from build123d import *

# Parameters (mm, degrees)
SZKIC2_W                    = 77
SZKIC2_H                    = 50
DODANIE_WYCI_GNI_CIE2_DEPTH = 4
SZKIC4_W                    = 50
SZKIC4_H                    = 46
WYTNIJ_WYCI_GNI_CIE1_DEPTH  = 4
SZKIC5_W                    = 77
SZKIC5_H                    = 4
DODANIE_WYCI_GNI_CIE3_DEPTH = 26
WYTNIJ_WYCI_GNI_CIE2_REACH  = 70.251
SZKIC6_R                    = 2
ZAOKR_GLENIE1_R             = 3
DODANIE_WYCI_GNI_CIE4_DEPTH = 4
DODANIE_WYCI_GNI_CIE5_DEPTH = 4
WYTNIJ_WYCI_GNI_CIE5_REACH  = 56.838
SZKIC9_R                    = 2


with BuildPart() as part:
    # Szkic2 → Dodanie-wyciągnięcie2 (new body)
    with BuildSketch(Plane(origin=(0, 0, 0), x_dir=(1, 0, 0), z_dir=(0, 1, 0))):
        Rectangle(SZKIC2_W, SZKIC2_H)
    extrude(amount=DODANIE_WYCI_GNI_CIE2_DEPTH)

    # Szkic4 → Wytnij-wyciągnięcie1 (cut)
    with BuildSketch(Plane.XZ):
        with Locations((0, -2)):
            Rectangle(SZKIC4_W, SZKIC4_H)
    extrude(amount=-WYTNIJ_WYCI_GNI_CIE1_DEPTH, mode=Mode.SUBTRACT)

    # Szkic5 → Dodanie-wyciągnięcie3 (add)
    with BuildSketch(Plane.XZ):
        with Locations((0, 23)):
            Rectangle(SZKIC5_W, SZKIC5_H)
    extrude(amount=DODANIE_WYCI_GNI_CIE3_DEPTH)

    # Szkic6 → Wytnij-wyciągnięcie2 (cut, up to next)
    with BuildSketch(Plane.XY.offset(25), mode=Mode.PRIVATE) as wytnij_wyci_gni_cie2_sk1:
        with Locations((26.5, -11)):
            Circle(SZKIC6_R)
    wytnij_wyci_gni_cie2_tool1 = extrude(wytnij_wyci_gni_cie2_sk1.sketch, amount=-WYTNIJ_WYCI_GNI_CIE2_REACH, mode=Mode.PRIVATE) & part.part
    # Szkic6 → Wytnij-wyciągnięcie2 (cut, up to next)
    with BuildSketch(Plane.XY.offset(25), mode=Mode.PRIVATE) as wytnij_wyci_gni_cie2_sk2:
        with Locations((-26.5, -11)):
            Circle(SZKIC6_R)
    wytnij_wyci_gni_cie2_tool2 = extrude(wytnij_wyci_gni_cie2_sk2.sketch, amount=-WYTNIJ_WYCI_GNI_CIE2_REACH, mode=Mode.PRIVATE) & part.part
    add(wytnij_wyci_gni_cie2_tool1.solids().sort_by_distance((26.5, -11, 25))[0], mode=Mode.SUBTRACT)
    add(wytnij_wyci_gni_cie2_tool2.solids().sort_by_distance((-26.5, -11, 25))[0], mode=Mode.SUBTRACT)

    # Zaokrąglenie1
    zaokr_glenie1_edges = [part.edges().sort_by_distance(p)[0] for p in [
        (-38.5, 2, -25),
        (38.5, 2, -25),
    ]]
    fillet(zaokr_glenie1_edges, radius=ZAOKR_GLENIE1_R)

    # Szkic7 → Dodanie-wyciągnięcie4 (add)
    with BuildSketch(Plane.ZY.offset(38.5)):
        Polygon((21, -26), (21, 0), (-22, 0), align=None)
    extrude(amount=-DODANIE_WYCI_GNI_CIE4_DEPTH)

    # Szkic8 → Dodanie-wyciągnięcie5 (add)
    with BuildSketch(Plane(origin=(38.5, 0, 0), x_dir=(0, 0, -1), z_dir=(1, 0, 0))):
        Polygon((-21, -26), (22, 0), (-21, 0), align=None)
    extrude(amount=-DODANIE_WYCI_GNI_CIE5_DEPTH)

    # Szkic9 → Wytnij-wyciągnięcie5 (cut, up to next)
    with BuildSketch(Plane(origin=(0, 4, 0), x_dir=(1, 0, 0), z_dir=(0, 1, 0)), mode=Mode.PRIVATE) as wytnij_wyci_gni_cie5_sk1:
        with Locations(Location((-30, 15, 0), (0, 0, 270))):
            Circle(SZKIC9_R)
    wytnij_wyci_gni_cie5_tool1 = extrude(wytnij_wyci_gni_cie5_sk1.sketch, amount=-WYTNIJ_WYCI_GNI_CIE5_REACH, mode=Mode.PRIVATE) & part.part
    # Szkic9 → Wytnij-wyciągnięcie5 (cut, up to next)
    with BuildSketch(Plane(origin=(0, 4, 0), x_dir=(1, 0, 0), z_dir=(0, 1, 0)), mode=Mode.PRIVATE) as wytnij_wyci_gni_cie5_sk2:
        with Locations(Location((-30, -15, 0), (0, 0, 270))):
            Circle(SZKIC9_R)
    wytnij_wyci_gni_cie5_tool2 = extrude(wytnij_wyci_gni_cie5_sk2.sketch, amount=-WYTNIJ_WYCI_GNI_CIE5_REACH, mode=Mode.PRIVATE) & part.part
    # Szkic9 → Wytnij-wyciągnięcie5 (cut, up to next)
    with BuildSketch(Plane(origin=(0, 4, 0), x_dir=(1, 0, 0), z_dir=(0, 1, 0)), mode=Mode.PRIVATE) as wytnij_wyci_gni_cie5_sk3:
        with Locations(Location((30, 15, 0), (0, 0, 270))):
            Circle(SZKIC9_R)
    wytnij_wyci_gni_cie5_tool3 = extrude(wytnij_wyci_gni_cie5_sk3.sketch, amount=-WYTNIJ_WYCI_GNI_CIE5_REACH, mode=Mode.PRIVATE) & part.part
    # Szkic9 → Wytnij-wyciągnięcie5 (cut, up to next)
    with BuildSketch(Plane(origin=(0, 4, 0), x_dir=(1, 0, 0), z_dir=(0, 1, 0)), mode=Mode.PRIVATE) as wytnij_wyci_gni_cie5_sk4:
        with Locations(Location((30, -15, 0), (0, 0, 270))):
            Circle(SZKIC9_R)
    wytnij_wyci_gni_cie5_tool4 = extrude(wytnij_wyci_gni_cie5_sk4.sketch, amount=-WYTNIJ_WYCI_GNI_CIE5_REACH, mode=Mode.PRIVATE) & part.part
    add(wytnij_wyci_gni_cie5_tool1.solids().sort_by_distance((-30, 4, -15))[0], mode=Mode.SUBTRACT)
    add(wytnij_wyci_gni_cie5_tool2.solids().sort_by_distance((-30, 4, 15))[0], mode=Mode.SUBTRACT)
    add(wytnij_wyci_gni_cie5_tool3.solids().sort_by_distance((30, 4, -15))[0], mode=Mode.SUBTRACT)
    add(wytnij_wyci_gni_cie5_tool4.solids().sort_by_distance((30, 4, 15))[0], mode=Mode.SUBTRACT)


solid = part.part
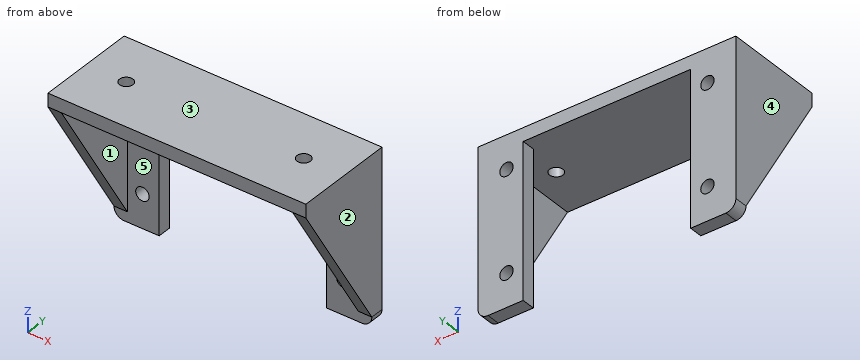
Part model, mm, in its own coordinate system. Face numbers are marked on the shaded views. A direction names the side the tool comes from. Coordinates: 2 decimals unless noted, no trailing zeros. Loops run counter-clockwise (first coordinate to the right, second up) from the corner with the lowest first, then second, coordinate; pieces in that order, holes last. Notation, with made-up numbers: (61, 21.25) - (83, 21.25) arc R23 cw to (83, 43.25) - close; hole circle Ø10 at (-6, 69.5). An arc over 180 degrees is marked (long way). Write each question's results on one line, items separated by ' | '. Start each with the question number.
Q1. Two-plate mould, pull along X, no slides. Class the marked faces 1, 2 and 3: +X half, -X half, draft (parallel to the pull), parting line (faces both ways), or undercut.
Q2. Drop flat-ended pins along their axis: pin 1 Ø4.5 at (x, z) = (30, 15) entering from -Y; pin 2 Ø5 at (x, y) = (-26.5, -11) entering from -Z; pin 3 Ø10 at (x, z) = (-30, -16.5) entering from -Y. Give the stop position or say it passes through.
Q3. Slice it at D-D on y = -11. Give the cut face in (x, z).
Q4. Which spindle directions (+Z, -Z, +X, -X, +Y, -Y) get a long thin tool onto all of the face, cutting with end or side? Do the marked faces 4 and 5. Say none if no direction does.
Q5. Probe line 1 along X through (y, z) = (1.95, -15); line 2 along Z through (x, y) = (29, 0.5); line 3 along X through (y, z) = (-2, 19). List the from-to ranges inside material, lowest first.
Q6. Slice it at C-C on x = 26.5. Give the cut face in (y, z).
Q7. Slice it at A-A on z = -21. Give the cut face in (x, y).
Q8. Slice it at B-B on x = -30. Give the cut face in (y, z).
Answer:
1) face 1: undercut | face 2: +X half | face 3: draft
2) pin 1: stops at y = 0 | pin 2: stops at z = 21 | pin 3: stops at y = -4.64
3) outline: (-38.5, -3.81) - (-34.5, -3.81) - (-34.5, 21) - (-28.5, 21) - (-28.5, 25) - (-38.5, 25) - close; (-24.5, 21) - (24.5, 21) - (24.5, 25) - (-24.5, 25) - close; (28.5, 21) - (34.5, 21) - (34.5, -3.81) - (38.5, -3.81) - (38.5, 25) - (28.5, 25) - close
4) face 4: +Z, -Z, -X, +Y, -Y | face 5: -Z, -Y
5) line 1: x = -38.5 to -32, -28 to -25, 25 to 28, 32 to 38.5 | line 2: z = -25 to -16.73, -13.27 to 13.27, 16.73 to 25 | line 3: x = -38.5 to -34.5, 34.5 to 38.5
6) outline: (-26, 21) - (-13, 21) - (-13, 25) - (-26, 25) - close; (-9, 21) - (0, 21) - (0, -25) - (4, -25) - (4, 25) - (-9, 25) - close
7) outline: (-38.5, -0.6) - (-34.5, -0.6) - (-34.5, 0) - (-25, 0) - (-25, 4) - (-38.5, 4) - close; (25, 0) - (34.5, 0) - (34.5, -0.6) - (38.5, -0.6) - (38.5, 4) - (25, 4) - close
8) outline: (-26, 21) - (0, 21) - (0, 17) - (4, 17) - (4, 25) - (-26, 25) - close; (0, -25) - (4, -25) - (4, -17) - (0, -17) - close; (0, -13) - (4, -13) - (4, 13) - (0, 13) - close
